from build123d import *

# Parameters (mm, degrees)
CUT_EXTRUDE_1_REACH      = 84.274
SKETCH_2_R               = 9
SKETCH_5_R               = 4.5
PATTERN_CIRCULAR_1_COUNT = 6
PATTERN_CIRCULAR_2_COUNT = 6
CHAMFER_1_SIZE           = 2
CHAMFER_2_SIZE           = 3
CHAMFER_3_SIZE           = 0.5


with BuildPart() as part:
    # Sketch 1 → Revolve 1 (revolve)
    with BuildSketch(Plane.XY, mode=Mode.PRIVATE) as revolve_1_sk:
        Polygon((0, 0), (0, 25), (28.29, 25), (28.29, 22), (38.29, 22), (38.29, 15), (66.29, 15), (66.29, 22), (74.29, 22), (74.29, 0), align=None)
    revolve(revolve_1_sk.sketch.rotate(Axis((-39.205856293, 0, 0), (1, 0, 0)), 90), axis=Axis((-39.205856293, 0, 0), (1, 0, 0)))

    # Sketch 2 → Cut-Extrude 1 (cut, up to next)
    with BuildSketch(Plane(origin=(74.29, 0, 0), x_dir=(0, 0, -1), z_dir=(1, 0, 0)), mode=Mode.PRIVATE) as cut_extrude_1_sk1:
        Circle(SKETCH_2_R)
    cut_extrude_1_tool1 = extrude(cut_extrude_1_sk1.sketch, amount=-CUT_EXTRUDE_1_REACH, mode=Mode.PRIVATE) & part.part
    add(cut_extrude_1_tool1.solids().sort_by_distance((74.29, 0, 0))[0], mode=Mode.SUBTRACT)

    # Sketch 3 → Hole Wizard 1 (revolve, cut)
    with BuildSketch(Plane(origin=(66.29, 16.75, 0), x_dir=(0, 0, 1), z_dir=(0, 1, 0))):
        Polygon((0, 0), (0, 8), (1.7, 8), (1.7, 5), (4.5, 5), (4.5, 0), align=None)
    hole_wizard_1 = revolve(axis=Axis((59.94, 16.75, 0), (1, 0, 0)), mode=Mode.SUBTRACT)

    # Sweep 2: sweep along a path in Sketch 6
    with BuildLine(Plane.XY) as sweep_2_path:
        ThreePointArc((66.29, 16.75), (51.18385823, 21.830048172), (42.216910691, 35.005641534))
    # Sketch 5 → Sweep 2 (sweep, cut)
    with BuildSketch(Plane.ZY.offset(-66.29)):
        with Locations((0, 16.75)):
            Circle(SKETCH_5_R)
    sweep_2 = sweep(path=sweep_2_path.line, mode=Mode.SUBTRACT)

    # Pattern Circular 1: Hole Wizard 1, Sweep 2 ×6 about axis
    pattern_circular_1_axis = Axis((0, 0, 0), (1, 0, 0))
    add([hole_wizard_1.rotate(pattern_circular_1_axis, i * 360 / PATTERN_CIRCULAR_1_COUNT) for i in range(1, PATTERN_CIRCULAR_1_COUNT)], mode=Mode.SUBTRACT)
    add([sweep_2.rotate(pattern_circular_1_axis, i * 360 / PATTERN_CIRCULAR_1_COUNT) for i in range(1, PATTERN_CIRCULAR_1_COUNT)], mode=Mode.SUBTRACT)

    # Sketch 9 → Hole Wizard M4 _1 (revolve, cut)
    with BuildSketch(Plane.ZX.offset(17.5)):
        Polygon((0, 0), (0, 7.591420021), (1.65, 6.6), (1.65, 0), align=None)
    hole_wizard_m4_1 = revolve(axis=Axis((-6.35, 17.5, 0), (1, 0, 0)), mode=Mode.SUBTRACT)

    # Pattern Circular 2: Hole Wizard M4 _1 ×6 about axis
    pattern_circular_2_axis = Axis((0, 0, 0), (1, 0, 0))
    for i in range(1, PATTERN_CIRCULAR_2_COUNT):
        add(hole_wizard_m4_1.rotate(pattern_circular_2_axis, i * 360 / PATTERN_CIRCULAR_2_COUNT), mode=Mode.SUBTRACT)

    # Chamfer 1
    chamfer_1_edges = [part.edges().sort_by_distance(p)[0] for p in [
        (28.29, 0, -25),
    ]]
    chamfer(chamfer_1_edges, length=CHAMFER_1_SIZE)

    # Chamfer 2
    chamfer_2_edges = [part.edges().sort_by_distance(p)[0] for p in [
        (38.29, 0, -22),
    ]]
    chamfer(chamfer_2_edges, length=CHAMFER_2_SIZE)

    # Chamfer 3
    chamfer_3_edges = [part.edges().sort_by_distance(p)[0] for p in [
        (66.29, 0, -22),
    ]]
    chamfer(chamfer_3_edges, length=CHAMFER_3_SIZE)


solid = part.part
Design review of the part built by this model. Coordinates are the model's own, in mm. A direction names the side the tool comes from. Give positions to 0.01 mm unless a question says otherwise; leave off trailing zeros. Write each loop counter-clockwise with the first axis right and the second up, starting at its lowest first coordinate (ties: lowest second). Pieces come first, ordered by that corner, then holes. Notation, with made-up numbers: M 28,19 L 41,19 A11 ccw 41,23 Z; hole C 26.5,23.25 d6. An arc over 180 degrees is marked long. Answer as a JSON object with one key per item and string values. Group by question number.
1) Mouldability with a two-part tool opening along Y and no side actions: class faces 1 (the face through (38.144, 11.65, -15.193)), 2 (the face through (3.25, 7.29, 14.39)), 3 (the face through (74.29, -0.3, 9.5)) as released by +Y, released by -Y, zero draft, split by the parting line, or undercut.
2) For line 1 along Y through (x, z) = (72.8, 0); line 2 along X through (y, z) = (5, 16); line 3 along Z through (x, y) = (2, -8), list the stretches that pass through material, from the lowest coordinate up.
3) We need section B-B (x = 41.5). Give the boundary of the cut face in (y, z).
4) Clearance check with flat-ended pins moving along their axes: pin 1 Ø6 at (x, y) = (28, -12) entering from -Z; pin 2 Ø10 at (x, y) = (44.5, 13.5) entering from +Z; pin 3 Ø5 at (x, y) = (8, -3) entering from +Z (3 decimals). State where each tip first meets the part, or that it passes through.
5) Tool access review of faces 4 (the face through (71.29, -19, 0)), 5 (the face through (72.769, -8.45, -16.204)), 6 (the face through (13.329, -7.509, 23.846)), 7 (the face through (3.25, -16.11, -0.89)), 8 (the face through (0, 11, 0)): name each direction out of +Z, -Z, +X, -X, +Y, -Y from which nothing blocks a thin tool from reaching the whole face with its end or side.
6) We need section A-A (x = 20.5). Give the boundary of the cut face in (y, z).
Answer key:
{
 "1": {"face 1": "split by the parting line", "face 2": "undercut", "face 3": "zero draft"},
 "2": {"line 1": "y = -22 to -18.45, -15.05 to -9, 9 to 15.05, 18.45 to 22", "line 2": "x = 0 to 38.29, 71.29 to 74.29", "line 3": "z = -23.69 to -16.63, -13.69 to -4.12, 4.12 to 13.69, 16.63 to 23.69"},
 "3": {"outline": "C 0,0 d30; hole C 0,0 d18"},
 "4": {"pin 1": "stops at z = -23.11", "pin 2": "stops at z = 12.36", "pin 3": "stops at z = 24.995"},
 "5": {"face 4": "none", "face 5": "+X", "face 6": "+X, -X", "face 7": "-X", "face 8": "+Z, -Z, -X, +Y, -Y"},
 "6": {"outline": "C 0,0 d50; hole C 0,0 d18"}
}
